Model file for the job. Use its own axes, mm. Face numbers are marked on the shaded views. A direction names the side the tool comes from. Give positions to 0.01 mm unless a question says otherwise; leave off trailing zeros. Loops run counter-clockwise (first coordinate to the right, second up) from the corner with the lowest first, then second, coordinate; pieces in that order, holes last. Notation, with made-up numbers: (34, 30) - (58, 30) arc R22 ccw to (58, 47) - close; hole circle Ø7 at (-10.5, -9). An arc over 180 degrees is marked (long way). Use a Markdown table: item, result.
from build123d import *

# Parameters (mm, degrees)
EXTRUDE1_DEPTH     = 100
CUT_EXTRUDE1_DEPTH = 100.461524227


with BuildPart() as part:
    # Sketch1 → Extrude1 (new body)
    with BuildSketch(Plane(origin=(0, 0, 0), x_dir=(1, 0, 0), z_dir=(0, 1, 0))):
        Polygon((0, 0), (30, -51.961524227), (-52.27241336, -99.461524227), (-82.27241336, -47.5), align=None)
    extrude(amount=EXTRUDE1_DEPTH)

    # Sketch2 → Cut-Extrude1 (cut, through all)
    with BuildSketch(Plane.XY):
        Polygon((-42.27241336, 78.639610307), (-10.452608206, 46.819805153), (-42.27241336, 15), (-74.092218513, 46.819805153), align=None)
    extrude(amount=CUT_EXTRUDE1_DEPTH, mode=Mode.SUBTRACT)


solid = part.part
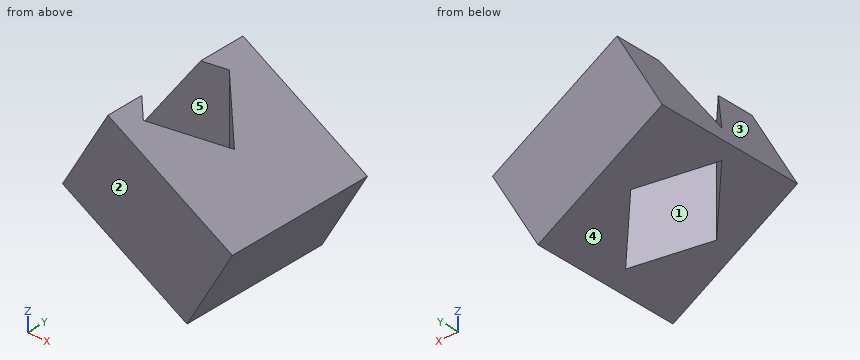
(1) Slice it at D-D, the plane y = 43. Write the cut outline in (x, z).
Computed:
| item | result |
|---|---|
| outline | (-82.27, 47.5) - (-70.27, 40.57) - (-70.27, 68.28) - close; (-14.27, 8.24) - (0, 0) - (30, 51.96) - (-14.27, 77.52) - close |
(2) Drill centre lines: probe 1 along Y at (x, z) = (-28.5, 25); probe 2 along Y at (x, z) = (-56, 56); probe 3 along X at (y, z) = (60, 62). Where is each one in solid material? Low to high. Write a range as [from, to].
Computed:
| item | result |
|---|---|
| probe 1 | [0, 28.77], [64.87, 100] |
| probe 2 | [0, 28.73], [64.91, 100] |
| probe 3 | [-73.9, -60.91], [-23.63, 12.61] |
(3) 3-axis set-ups, long thin cutter, end or side, ignore diameter. For the marked faces 4 and 5: which of +Z, -Z, +X, -X, +Y, -Y reach the whole face in a straight line?
Computed:
| item | result |
|---|---|
| face 4 | -Z, -X, +Y, -Y |
| face 5 | +Z, -Z |
(4) Mould opens along Y. For the marked faces 1, 2 and 3 say: pulls with the +Y half, pulls with the -Y half, needs draft (parallel to the pull), parting line crosses it, or undercut.
Computed:
| item | result |
|---|---|
| face 1 | undercut |
| face 2 | pulls with the -Y half |
| face 3 | needs draft |
(5) Slice it at A-A, the plane y = 76. Write the cut outline in (x, z).
Computed:
| item | result |
|---|---|
| outline | (-82.27, 47.5) - (-44.91, 25.93) - (-44.91, 95.21) - (-52.27, 99.46) - close; (-39.63, 22.88) - (0, 0) - (30, 51.96) - (-39.63, 92.16) - close |
(6) Slice it at C-C, the plane z = 45.5. Write the cut outline in (x, y).
Computed:
| item | result |
|---|---|
| outline | (-78.81, 0) - (26.27, 0) - (26.27, 100) - (-78.81, 100) - close; hole (-74.09, 46.82) - (-42.27, 15) - (-10.45, 46.82) - (-42.27, 78.64) - close |
(7) Pin check, flat tips, straight feed: P1, Ø6, axis at y = 64.5, z = 42, coming from the -X side; P2, Ø1.5, axis at x = -4.5, y = 31, coming from the -Z side; P3, Ø4, axis at y = 32.5, z = 31, coming from the +X side. Stop position of each tip, or through.
Computed:
| item | result |
|---|---|
| P1 | x = -77.94 |
| P2 | z = 2.17 |
| P3 | x = 19.05 |
(8) Slice it at B-B, the plane x = -60. Write the cut outline in (y, z), plus the area to 3 significant figures.
Computed:
| item | result |
|---|---|
| outline | (0, 34.64) - (32.73, 34.64) - (32.73, 86.08) - (0, 86.08) - close; (60.91, 34.64) - (100, 34.64) - (100, 86.08) - (60.91, 86.08) - close |
| area | 3,690 mm² |
